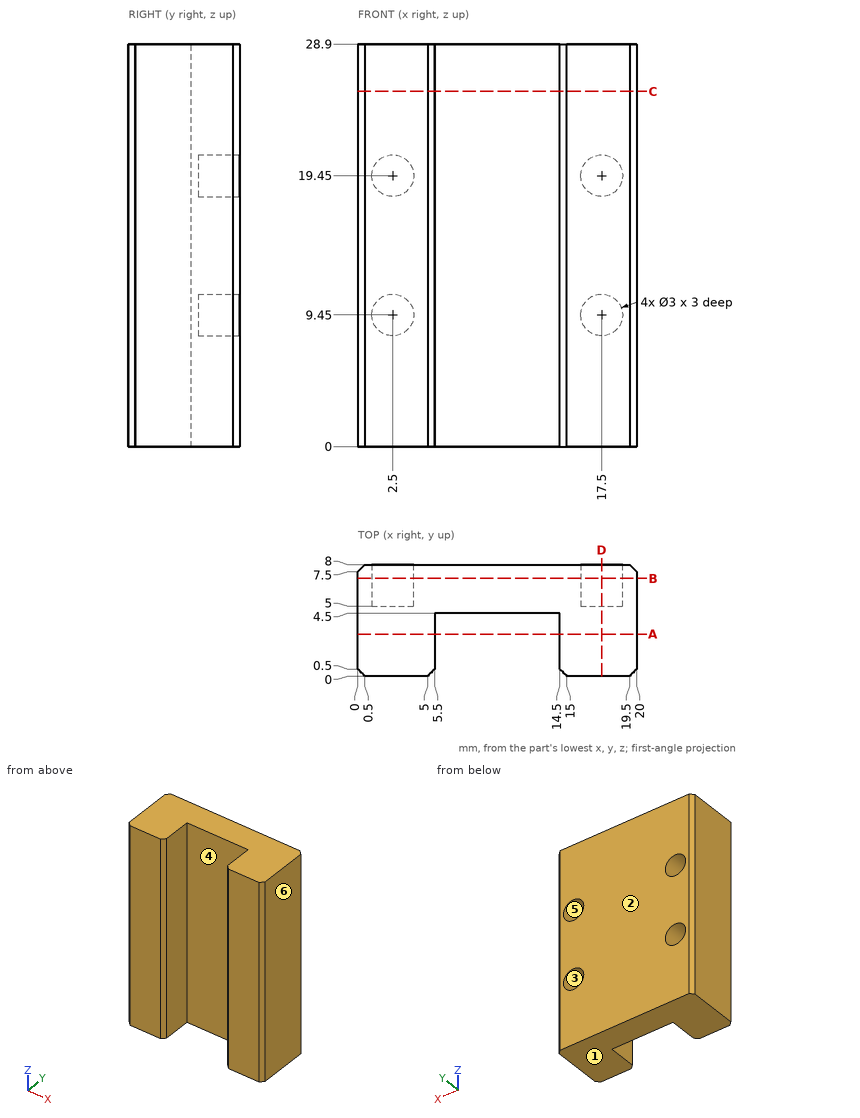
Could you check a few things on this drawing? It's one solid part, dimensions in mm from its lowest x, y, z. A direction names the side the tool comes from. Round coordinates to 2 decimals unless told otherwise and drop trailing zeros. Write each loop counter-clockwise with the first axis right and the second up, starting at its lowest first coordinate (ties: lowest second). Pieces come first, ordered by that corner, then holes. Notation, with made-up numbers: (43, 4) -> (84, 4) arc R22 ccw to (84, 20) -> close; hole circle Ø8 at (-5, 26.25). An arc over 180 degrees is marked (long way). Use one line per item in the form item = value. Start each with the question number.
Q1. I'm going to push flat-ended pins straight in: P1, Ø1.5, axis at x = 2, z = 9, coming from the +Y side; P2, Ø2.5, axis at x = 12, z = 17.5, coming from the -Y side. Where does each tip first touch, or does it pass through?
Q2. If I drill on probe 1 along Z at (x, y) = (2.5, 5.9); probe 2 along X at (y, z) = (1, 22); probe 3 along Z at (x, y) = (16.75, 6.75), over which ranges is the centre line in solid material (lowest first)? Write a range as [from, to].
Q3. We'd pull the mould along Z, two halves only. Please class the marked faces 1, 2 and 3: +Z half, -Z half, draft (parallel to the pull), parting line (faces both ways), or undercut.
Q4. Imagine slicing it at D-D (x = 17.5). Please give me the cut outline in (y, z).
Q5. Imagine slicing it at B-B (y = 7). Please give me the cut outline in (x, z).
Q6. Imagine slicing it at A-A (y = 3). Please give me the cut outline in (x, z).
Q7. Imagine slicing it at C-C (z = 25.5). Please give me the cut outline in (x, y).
Q8. Which directions (+Z, -Z, +X, -X, +Y, -Y) give clear straight access to the entire face, cutting with the end or side of a thin tool? Please do the marked faces 4, 5 and 6.
Worked out:
q1.P1 = 5
q1.P2 = 4.5
q2.probe_1 = [0, 7.95], [10.95, 17.95], [20.95, 28.9]
q2.probe_2 = [0, 5.5], [14.5, 20]
q2.probe_3 = [0, 8.15], [10.75, 18.15], [20.75, 28.9]
q3.face_1 = -Z half
q3.face_2 = draft
q3.face_3 = undercut
q4.outline = (0, 0) -> (8, 0) -> (8, 7.95) -> (5, 7.95) -> (5, 10.95) -> (8, 10.95) -> (8, 17.95) -> (5, 17.95) -> (5, 20.95) -> (8, 20.95) -> (8, 28.9) -> (0, 28.9) -> close
q5.outline = (0, 0) -> (20, 0) -> (20, 28.9) -> (0, 28.9) -> close; hole circle Ø3 at (2.5, 9.45); hole circle Ø3 at (2.5, 19.45); hole circle Ø3 at (17.5, 9.45); hole circle Ø3 at (17.5, 19.45)
q6.outline = (0, 0) -> (5.5, 0) -> (5.5, 28.9) -> (0, 28.9) -> close; (14.5, 0) -> (20, 0) -> (20, 28.9) -> (14.5, 28.9) -> close
q7.outline = (0, 0.5) -> (0.5, 0) -> (5, 0) -> (5.5, 0.5) -> (5.5, 4.5) -> (14.5, 4.5) -> (14.5, 0.5) -> (15, 0) -> (19.5, 0) -> (20, 0.5) -> (20, 7.5) -> (19.5, 8) -> (0.5, 8) -> (0, 7.5) -> close
q8.face_4 = +Z, -Z, -Y
q8.face_5 = +Y
q8.face_6 = +Z, -Z, +X, +Y, -Y
